```python
from build123d import *

# Parameters (mm, degrees)
F2_W          = 40
F2_H          = 25.9671732676
F3_DEPTH      = 19.376
F3_DEPTH_BACK = 19.376
F4_DEPTH      = 19.376
F4_DEPTH_BACK = 19.376


with BuildPart() as f1:
    # F0 (on Front) → F1 (revolve)
    with BuildSketch(Plane.XZ):
        with BuildLine():
            Line((-18, 19), (-19.375, 0))
            Line((-19.375, 0), (-16.3671544762, 0))
            Line((-16.3671544762, 0), (-14.9921544762, 19))
            Line((-14.9921544762, 19), (-2.5980762114, 40.4671732676))
            ThreePointArc((-2.5980762114, 40.4671732676), (-1.5, 41.565249479), (0, 41.9671732676))
            Line((0, 41.9671732676), (0, 44.9671732676))
            ThreePointArc((0, 44.9671732676), (-11.8033499729, 40.3259888916), (-17.2843902722, 28.8884253296))
            Line((-17.2843902722, 28.8884253296), (-18, 19))
        make_face()
    revolve(axis=Axis((0, 0, 30.4835866338), (0, 0, 1)))

    # F2 (on Right) → F3 (cut, two sides)
    with BuildSketch(Plane.YZ) as f3_sk:
        with Locations((-25, 31.9835866338)):
            Rectangle(F2_W, F2_H)
        with Locations((25, 31.9835866338)):
            Rectangle(F2_W, F2_H)
    extrude(amount=F3_DEPTH, mode=Mode.SUBTRACT)
    extrude(f3_sk.sketch, amount=-F3_DEPTH_BACK, mode=Mode.SUBTRACT)

    # F0 (on Front) → F4 (cut, two sides)
    with BuildSketch(Plane.XZ) as f4_sk:
        with BuildLine():
            Line((-2.5980762114, 40.4671732676), (-14.9921544762, 19))
            Line((-14.9921544762, 19), (0, 19))
            Line((0, 19), (0, 41.9671732676))
            ThreePointArc((0, 41.9671732676), (-1.5, 41.565249479), (-2.5980762114, 40.4671732676))
        make_face()
        with BuildLine():
            Line((0, 41.9671732676), (0, 19))
            Line((0, 19), (14.9921544762, 19))
            Line((14.9921544762, 19), (2.5980762114, 40.4671732676))
            ThreePointArc((2.5980762114, 40.4671732676), (1.5, 41.565249479), (0, 41.9671732676))
        make_face()
    extrude(amount=-F4_DEPTH, mode=Mode.SUBTRACT)
    extrude(f4_sk.sketch, amount=F4_DEPTH_BACK, mode=Mode.SUBTRACT)


solid = f1.part
```
Work out the finished part from the listing and answer in its coordinate system (mm). A direction names the side the tool comes from. Round coordinates to 2 decimals unless told otherwise and drop trailing zeros. Order: outer loops, then holes, each group sorted by start corner. A loop starts at its lowest first (then second) coordinate and runs counter-clockwise, first axis right, second up.
Q1. Given pin 1 Ø1.5 at (x, z) = (-11, 29) entering from -Y; pin 2 Ø3 at (y, z) = (-4, 38.5) entering from -X; pin 3 Ø12 at (x, y) = (-7.5, 4) entering from +Z; pin 4 Ø12.5 at (x, z) = (0, 32) entering from -Y, each flat-ended and moving along its own axis, determine where each tip first touches the part or whether it passes through.
Solution:
pin 1: stops at y = -5
pin 2: stops at x = -14.1
pin 3: stops at z = 44.79
pin 4: passes through
Q2. Find the intervals of material crossed by line 1 along X through (y, z) = (-0.5, 21); line 2 along Z through (x, y) = (-13.5, -11.5); line 3 along Y through (x, z) = (-13, 17), in increasing order.
Solution:
line 1: x = -17.85 to -13.84, 13.84 to 17.85
line 2: z = 0 to 19
line 3: y = -12.66 to -7.75, 7.75 to 12.66
Q3. A cutting plane is placed at C-C, the plane x = 13.5. Count the separate pieces of the cut face and the enclosed holes in it, then the cut area to 3 significant figures.
Solution:
separate pieces: 3
enclosed holes: 0
area: 354 mm2
Q4. The mould has two halves that part along X. Classify faces 1 (the conical face through (2.02, -15.385, 11.744)), 2 (the flat face through (7, -5, 34)), 3 (the conical face through (18.56, -0.82, 11.03)): pulls with the +X half, pulls with the -X half, needs draft (parallel to the pull), parting line crosses it, or undercut.
Solution:
face 1: undercut
face 2: needs draft
face 3: parting line crosses it
Q5. A cutting plane is placed at A-A, the plane x = 0. Determine the outline of the cut face in (y, z) (3 decimals).
Solution:
outline: (-19.375, 0) - (-16.367, 0) - (-14.992, 19) - (-18, 19) - close; (-5, 41.967) - (5, 41.967) - (5, 44.23) arc R17.33 ccw to (-5, 44.23) - close; (14.992, 19) - (16.367, 0) - (19.375, 0) - (18, 19) - close
Q6. A tool of negligible diameter and unlimited length cuts with its end or side. For faces 4 (the cylindrical face through (0.044, -0.07, 41.967)), 5 (the flat face through (-7, 5, 34)), from which of +Z, -Z, +X, -X, +Y, -Y can it reach the whole face along a straight path? Write none if from no direction.
Solution:
face 4: -Z, +Y, -Y
face 5: +Z, +X, -X, +Y
Q7. A cutting plane is placed at B-B, the plane z = 25. Determine the outline of the cut face in (x, y), then the cut area to 3 significant figures.
Solution:
outline: (-16.84, -5) - (-11.53, -5) - (-11.53, 5) - (-16.84, 5) arc R17.57 ccw to start; (11.53, -5) - (16.84, -5) arc R17.57 ccw to (16.84, 5) - (11.53, 5) - close
area: 116 mm2
Q8. A cutting plane is placed at D-D, the plane z = 12.5. Determine the outline of the cut face in (x, y), then the cut area to 3 significant figures.
Solution:
outline: circle Ø36.94 at (0, 0); hole circle Ø30.93 at (0, 0)
area: 321 mm2
